from build123d import *

# Parameters (mm, degrees)
F1_DEPTH = 3.175
F2_W     = 8.9662
F2_H     = 11.43
F2_W_2   = 12.764952
F2_H_2   = 4.638044
F2_R     = 2.150647
F2_W_3   = 10.33394
F2_H_3   = 4.94447
F3_DEPTH = 25.4


with BuildPart() as f1:
    # F0 (on Front) → F1 (new body)
    with BuildSketch(Plane.XZ):
        with BuildLine():
            ThreePointArc((63.5, 22.225), (61.640128, 26.715128), (57.15, 28.575))
            Line((57.15, 28.575), (-57.15, 28.575))
            ThreePointArc((-57.15, 28.575), (-61.640128, 26.715128), (-63.5, 22.225))
            Line((-63.5, 22.225), (-63.5, -22.225))
            ThreePointArc((-63.5, -22.225), (-61.640128, -26.715128), (-57.15, -28.575))
            Line((-57.15, -28.575), (57.15, -28.575))
            ThreePointArc((57.15, -28.575), (61.640128, -26.715128), (63.5, -22.225))
            Line((63.5, -22.225), (63.5, 22.225))
        make_face()
    extrude(amount=F1_DEPTH)

    # F2 (on face) → F3 (cut)
    with BuildSketch(Plane.XZ.offset(3.175)):
        with Locations((-44.2849, -14.605)):
            Rectangle(F2_W, F2_H)
        with Locations((-21.180364, -18.000978)):
            Rectangle(F2_W_2, F2_H_2)
        with Locations((-4.65206, -16.583629)):
            Circle(F2_R)
        with Locations((3.967021, -16.501367)):
            Circle(F2_R)
        with Locations((12.624987, -16.556866)):
            Circle(F2_R)
        with Locations((38.731862, -17.752491)):
            Rectangle(F2_W_3, F2_H_3)
    extrude(amount=-F3_DEPTH, mode=Mode.SUBTRACT)


solid = f1.part
Design review of the part built by this model. Coordinates are the model's own, in mm. A direction names the side the tool comes from. Coordinates: 2 decimals unless noted, no trailing zeros. Order: outer loops, then holes, each group sorted by start corner. A loop starts at its lowest first (then second) coordinate and runs counter-clockwise, first axis right, second up.
Item 1: For pin 1 Ø2 at (x, z) = (-33, 20.5) entering from +Y; pin 2 Ø3.5 at (x, z) = (12.62, -16.56) entering from +Y, all flat-tipped, find the tip position at first contact; note any pin that passes through.
Item 2: Take a section at A-A, the plane y = -1.2. Write out the cut boundary in (x, z) (3 decimals).
Item 3: For line 1 (Z direction, x = -18.5, y = -2.2) (3 decimals); line 2 (Z direction, x = -41.5, y = -1.2) (3 decimals); line 3 (X direction, y = -1.9, z = -10), list the stretches that pass through material, from the lowest coordinate up.
Item 4: The part is to be moulded in two halves that separate along Y. For faces 3 (the flat face through (-21, -2, -15.682)), 4 (the flat face through (-1, -3.175, 0)), say which applies: pulls with the +Y half, pulls with the -Y half, needs draft (parallel to the pull), parting line crosses it, or undercut.
Item 5: For faces 1 (the flat face through (39, -2, -15.28)), 2 (the cylindrical face through (-61.689, -1.565, -26.665)), list the 3-axis set-ups (+Z, -Z, +X, -X, +Y, -Y) from which the entire face can be reached by the end or side of a thin tool; tool diameter is ignored.
The answers:
1. pin 1: stops at y = 0
1. pin 2: passes through
2. outline: (-63.5, -22.225) arc R6.35 ccw to (-57.15, -28.575) - (57.15, -28.575) arc R6.35 ccw to (63.5, -22.225) - (63.5, 22.225) arc R6.35 ccw to (57.15, 28.575) - (-57.15, 28.575) arc R6.35 ccw to (-63.5, 22.225) - close; hole (-48.768, -20.32) - (-39.802, -20.32) - (-39.802, -8.89) - (-48.768, -8.89) - close; hole (-27.563, -20.32) - (-14.798, -20.32) - (-14.798, -15.682) - (-27.563, -15.682) - close; hole circle Ø4.301 at (-4.652, -16.584); hole circle Ø4.301 at (3.967, -16.501); hole circle Ø4.301 at (12.625, -16.557); hole (33.565, -20.225) - (43.899, -20.225) - (43.899, -15.28) - (33.565, -15.28) - close
3. line 1: z = -28.575 to -20.32, -15.682 to 28.575
3. line 2: z = -28.575 to -20.32, -8.89 to 28.575
3. line 3: x = -63.5 to -48.77, -39.8 to 63.5
4. face 3: needs draft
4. face 4: pulls with the -Y half
5. face 1: +Y, -Y
5. face 2: -Z, -X, +Y, -Y
